Build history of the part. All positions in model axes, mm. A direction names the side the tool comes from. Round coordinates to 2 decimals unless told otherwise and drop trailing zeros. Order: outer loops, then holes, each group sorted by start corner. A loop starts at its lowest first (then second) coordinate and runs counter-clockwise, first axis right, second up. Notation, with made-up numbers: (21, 14.25) -> (37, 14.25) arc R14 cw to (37, 19.25) -> close; hole circle Ø9 at (0.25, 38). An arc over 180 degrees is marked (long way). Write item = value, one per line.
from build123d import *

# Parameters (mm, degrees)
SKETCH3_R           = 1.5
BOSS_EXTRUDE4_DEPTH = 2
SKETCH8_W           = 129
SKETCH8_H           = 9
BOSS_EXTRUDE5_DEPTH = 10
SKETCH10_W          = 5.5
SKETCH10_H          = 4.5
SKETCH10_W_2        = 4.80000148
SKETCH10_H_2        = 3.5999988
SKETCH10_H_3        = 3.597941299
SKETCH10_W_3        = 5.99999908
SKETCH10_H_4        = 4.00000054
CUT_EXTRUDE1_DEPTH  = 18
SKETCH11_W          = 8
SKETCH11_H          = 6.5
CUT_EXTRUDE2_DEPTH  = 4
SKETCH12_W          = 111
SKETCH12_H          = 8
CUT_EXTRUDE3_DEPTH  = 10


with BuildPart() as part:
    # Sketch3 → Boss-Extrude4 (new body)
    with BuildSketch(Plane(origin=(0, 0, 0), x_dir=(1, 0, 0), z_dir=(0, 1, 0))):
        Polygon((-64.5, -13), (64.5, -13), (64.5, 5), (54.5, 5), (54.5, -3), (-54.5, -3), (-54.5, 5), (-64.5, 5), align=None)
        with Locations((-59.5, 0)):
            Circle(SKETCH3_R, mode=Mode.SUBTRACT)
        with Locations((59.5, 0)):
            Circle(SKETCH3_R, mode=Mode.SUBTRACT)
    extrude(amount=BOSS_EXTRUDE4_DEPTH)

    # Sketch8 → Boss-Extrude5 (add)
    with BuildSketch(Plane(origin=(0, 2, 0), x_dir=(1, 0, 0), z_dir=(0, 1, 0))):
        with Locations((0, -8.5)):
            Rectangle(SKETCH8_W, SKETCH8_H)
    extrude(amount=-BOSS_EXTRUDE5_DEPTH)

    # Sketch10 → Cut-Extrude1 (cut)
    with BuildSketch(Plane.XY.offset(13)):
        with Locations((-52.513655094, -3.248549409)):
            Rectangle(SKETCH10_W, SKETCH10_H)
        with Locations((-29.513655374, -3.248549409)):
            Rectangle(SKETCH10_W, SKETCH10_H)
        with Locations((2.541347826, -1.898548299)):
            Rectangle(SKETCH10_W_2, SKETCH10_H_2)
        with Locations((10.541347066, -1.898548299)):
            Rectangle(SKETCH10_W_2, SKETCH10_H_2)
        with Locations((18.541346306, -1.898548299)):
            Rectangle(SKETCH10_W_2, SKETCH10_H_2)
        with Locations((26.541345546, -1.89957705)):
            Rectangle(SKETCH10_W_2, SKETCH10_H_3)
        with Locations((34.541344786, -2.098549169)):
            Rectangle(SKETCH10_W_3, SKETCH10_H_4)
        with Locations((42.541344026, -2.098549169)):
            Rectangle(SKETCH10_W_3, SKETCH10_H_4)
        with Locations((50.541343266, -1.898548299)):
            Rectangle(SKETCH10_W_2, SKETCH10_H_2)
    extrude(amount=-CUT_EXTRUDE1_DEPTH, mode=Mode.SUBTRACT)

    # Sketch11 → Cut-Extrude2 (cut)
    with BuildSketch(Plane.XY.offset(13)):
        with Locations((-52.513655094, -3.248549409)):
            Rectangle(SKETCH11_W, SKETCH11_H)
        with Locations((-29.513655374, -3.248549409)):
            Rectangle(SKETCH11_W, SKETCH11_H)
    extrude(amount=-CUT_EXTRUDE2_DEPTH, mode=Mode.SUBTRACT)

    # Sketch12 → Cut-Extrude3 (cut)
    with BuildSketch(Plane(origin=(0, 2, 0), x_dir=(1, 0, 0), z_dir=(0, 1, 0))):
        with Locations((0, 1)):
            Rectangle(SKETCH12_W, SKETCH12_H)
    extrude(amount=-CUT_EXTRUDE3_DEPTH, mode=Mode.SUBTRACT)


solid = part.part
Q1. Cut at A-A, the plane z = 0. List the corners of the cut face in (x, y).
Check values:
outline = (-64.5, 0) -> (-61, 0) -> (-61, 2) -> (-64.5, 2) -> close; (-58, 0) -> (-55.5, 0) -> (-55.5, 2) -> (-58, 2) -> close; (55.5, 0) -> (58, 0) -> (58, 2) -> (55.5, 2) -> close; (61, 0) -> (64.5, 0) -> (64.5, 2) -> (61, 2) -> close
Q2. Mould opens along Y. For faces 1 (the face through (-30, -0.999, 7)), 2 (the face through (-55.5, 1, -1)), 3 (the face through (-0.3, 0, 3.5)) say: released by +Y, released by -Y, zero draft, split by the parting line, or undercut.
Check values:
face_1 = undercut
face_2 = zero draft
face_3 = released by -Y
Q3. Cut at B-B, the plane x = -59.5. List the corners of the cut face in (y, z).
Check values:
outline = (-8, 4) -> (0, 4) -> (0, 1.5) -> (2, 1.5) -> (2, 13) -> (-8, 13) -> close; (0, -5) -> (2, -5) -> (2, -1.5) -> (0, -1.5) -> close
Q4. Which spindle directions (+Z, -Z, +X, -X, +Y, -Y) get a long thin tool onto all of the face, cutting with end or side? Do faces 4 (the face through (-30, -6.499, 11)), 5 (the face through (-30, -5.499, 7)), 6 (the face through (-1, -4, 4)). Say none if no direction does.
Check values:
face_4 = +Z
face_5 = +Z, -Z
face_6 = -Z, +X, -X, -Y
Q5. Probe probe 1 along X at (y, z) = (1.3, 0); probe 2 along X at (y, z) = (-4.75, 10.5); probe 3 along X at (y, z) = (-3.75, 5). List the from-to ranges inside material, lowest first.
Check values:
probe_1 = -64.5 to -61, -58 to -55.5, 55.5 to 58, 61 to 64.5
probe_2 = -64.5 to -56.51, -48.51 to -33.51, -25.51 to 64.5
probe_3 = -64.5 to -55.26, -49.76 to -32.26, -26.76 to 31.54, 37.54 to 39.54, 45.54 to 64.5
Q6. Cut at C-C, the plane z = 11.5. Give the number of separate pieces and of enclosed holes in the cut face, and give its area (3 significant figures).
Check values:
separate_pieces = 1
enclosed_holes = 9
area = 1,050 mm²
Q7. Flat gauge pins, fed straight in: pin 1 (6 mm diameter, centred on x = 44.5, y = -5.5, fed in from -Z); pin 2 (1 mm diameter, centred on y = -4, z = 3, fed in from -X); pin 3 (1 mm diameter, centred on x = -15, y = 1, fed in from -Z). Where does each tip first touch, or does it go through?
Check values:
pin_1 = 4
pin_2 = through
pin_3 = 3
